from build123d import *

# Parameters (mm, degrees)
ESQUISSE1_W                  = 80
ESQUISSE1_H                  = 80
BOSS_EXTRU_1_DEPTH           = 9
ESQUISSE2_R                  = 19.25
ESQUISSE2_R_2                = 2.25
ESQUISSE2_R_3                = 3.25
ENL_V_MAT_EXTRU_1_DEPTH      = 114.494493258
ENL_V_MAT_EXTRU_2_DEPTH      = 114.494493258
ENL_V_MAT_EXTRU_2_DEPTH_BACK = 114.494493258
ESQUISSE3_W                  = 30
ESQUISSE3_H                  = 8
CONG_1_R                     = 4


with BuildPart() as part:
    # Esquisse1 → Boss.-Extru.1 (new body)
    with BuildSketch(Plane.XY):
        with Locations((40, 40)):
            Rectangle(ESQUISSE1_W, ESQUISSE1_H)
    extrude(amount=BOSS_EXTRU_1_DEPTH)

    # Esquisse2 → Enlèv. mat.-Extru.1 (cut, through all)
    with BuildSketch(Plane.XY.offset(9)):
        with Locations((40, 40)):
            Circle(ESQUISSE2_R)
        with Locations((73.234018716, 40)):
            Circle(ESQUISSE2_R_2)
        with Locations((40, 73.234018716)):
            Circle(ESQUISSE2_R_2)
        with Locations(Location((6.765981284, 40, 0), (0, 0, 180))):
            Circle(ESQUISSE2_R_2)
        with Locations(Location((40, 6.765981284, 0), (0, 0, 180))):
            Circle(ESQUISSE2_R_2)
        with Locations((10, 65)):
            Circle(ESQUISSE2_R_3)
        with Locations(Location((70, 65, 0), (0, 0, 180))):
            Circle(ESQUISSE2_R_3)
        with Locations((70, 15)):
            Circle(ESQUISSE2_R_3)
        with Locations(Location((10, 15, 0), (0, 0, 180))):
            Circle(ESQUISSE2_R_3)
    extrude(amount=-ENL_V_MAT_EXTRU_1_DEPTH, mode=Mode.SUBTRACT)

    # Esquisse3 → Enlèv. mat.-Extru.2 (cut, two sides: drawn at the far end of the back side and taken through both)
    with BuildSketch(Plane.XY.offset(9).offset(-ENL_V_MAT_EXTRU_2_DEPTH_BACK)):
        with Locations((15, 76)):
            Rectangle(ESQUISSE3_W, ESQUISSE3_H)
        with Locations((65, 76)):
            Rectangle(ESQUISSE3_W, ESQUISSE3_H)
        with Locations((15, 4)):
            Rectangle(ESQUISSE3_W, ESQUISSE3_H)
        with Locations((65, 4)):
            Rectangle(ESQUISSE3_W, ESQUISSE3_H)
    extrude(amount=ENL_V_MAT_EXTRU_2_DEPTH + ENL_V_MAT_EXTRU_2_DEPTH_BACK, mode=Mode.SUBTRACT)

    # Congé1
    cong_1_edges = [part.edges().sort_by_distance(p)[0] for p in [
        (30, 72, 4.5),
        (50, 72, 4.5),
        (50, 8, 4.5),
        (30, 8, 4.5),
        (0, 8, 4.5),
        (30, 0, 4.5),
        (50, 0, 4.5),
        (80, 8, 4.5),
        (80, 72, 4.5),
        (50, 80, 4.5),
        (30, 80, 4.5),
        (0, 72, 4.5),
    ]]
    fillet(cong_1_edges, radius=CONG_1_R - 0.0001)  # a hair under: the kernel refuses the full size


solid = part.part
Work out the finished part from the listing and answer in its coordinate system (mm). A direction names the side the tool comes from. Round coordinates to 2 decimals unless told otherwise and drop trailing zeros. Loops run counter-clockwise (first coordinate to the right, second up) from the corner with the lowest first, then second, coordinate; pieces in that order, holes last. Notation, with made-up numbers: (1, 8.25) - (22, 8.25) arc R28 cw to (22, 29.25) - close; hole circle Ø5 at (9, 14.25). An arc over 180 degrees is marked (long way). Use one line per item in the form item = value. Start each with the question number.
(1) Find section B-B on x = 10. Determine the outline of the cut face in (y, z).
(2) Find section D-D on z = 4.25. Give the number of separate pieces and of enclosed holes in the cut face, and give its area (3 significant figures).
(3) Consider line 1 (Y direction, x = 70, z = 3.5); line 2 (Y direction, x = 40, z = 5.5); line 3 (Y direction, x = 13, z = 2.5). Determine where each line is inside the solid, lowest interval first.
(4) Which of the six approach directions +Z, -Z, +X, -X, +Y, -Y give full straight-line access (tool end or side, diameter ignored) to faces 1 (the face through (15, 8, 4)), 2 (the face through (31.141, 78.797, 4.563))?
(5) Find section A-A on y = 65. Determine the outline of the cut face in (x, z).
(6) Determine the mould class of faces 3 (the face through (1.141, 70.797, 4.563)), 4 (the face through (39.707, 75.465, 4.563)), 5 (the face through (31, 58, 0)) for opening direction X: +X half, -X half, draft (parallel to the pull), parting line (faces both ways), or undercut.
(7) Find section C-C on x = 58. Determine the outline of the cut face in (y, z), and give its area (3 significant figures).
Answer list:
q1.outline = (8, 0) - (11.75, 0) - (11.75, 9) - (8, 9) - close; (18.25, 0) - (61.75, 0) - (61.75, 9) - (18.25, 9) - close; (68.25, 0) - (72, 0) - (72, 9) - (68.25, 9) - close
q2.separate_pieces = 1
q2.enclosed_holes = 9
q2.area = 4,070 mm^2
q3.line_1 = 8 to 11.75, 18.25 to 61.75, 68.25 to 72
q3.line_2 = 0 to 4.52, 9.02 to 20.75, 59.25 to 70.98, 75.48 to 80
q3.line_3 = 8 to 13.75, 16.25 to 63.75, 66.25 to 72
q4.face_1 = +Z, -Z, -X, -Y
q4.face_2 = +Z, -Z, -X, +Y
q5.outline = (0, 0) - (6.75, 0) - (6.75, 9) - (0, 9) - close; (13.25, 0) - (66.75, 0) - (66.75, 9) - (13.25, 9) - close; (73.25, 0) - (80, 0) - (80, 9) - (73.25, 9) - close
q6.face_3 = -X half
q6.face_4 = undercut
q6.face_5 = draft
q7.outline = (8, 0) - (33.18, 0) - (33.18, 9) - (8, 9) - close; (46.82, 0) - (72, 0) - (72, 9) - (46.82, 9) - close
q7.area = 453 mm^2
